CAD build for the part. Positions are in the model's coordinates, mm. A direction names the side the tool comes from. Give positions to 0.01 mm unless a question says otherwise; leave off trailing zeros. Write each loop counter-clockwise with the first axis right and the second up, starting at its lowest first coordinate (ties: lowest second). Pieces come first, ordered by that corner, then holes. Notation, with made-up numbers: (8.25, 14.5) - (66.25, 14.5) arc R29 cw to (66.25, 46.5) - close; hole circle Ø7 at (10, -34). An arc over 180 degrees is marked (long way). Answer as a JSON object with one key per item and string values.
from build123d import *

# Parameters (mm, degrees)
FLANGE_BASE1_DEPTH    = 5
CORTE_EXTRUS_O1_REACH = 55.903
ESBO_O2_R             = 1
QUEBRA_CANTO1_START   = -5
QUEBRA_CANTO1_DEPTH   = 5


# Read off the part's stored shape, not the designer's step: Quebra-Canto1
# Sheet-metal steps are written as plain solids
with BuildPart() as part:
    # Esboço1 → Flange-base1 (new body)
    with BuildSketch(Plane.XY):
        Polygon((-7.191672609, 43.102851176), (1.806254311, 43.102851176), (1.806254311, 37.302851176), (0.606254311, 37.302851176), (0.606254311, 34.902851176), (1.806254311, 34.902851176), (1.806254311, 31.102851176), (4.806254311, 31.102851176), (4.806254311, 34.902851176), (6.006254311, 34.902851176), (6.006254311, 37.302851176), (4.806254311, 37.302851176), (4.806254311, 43.102851176), (13.804181231, 43.102851176), (13.804181231, 48.102851176), (23.804181231, 48.102851176), (23.804181231, -21.897149822), (13.804181231, -21.897149822), (13.804181231, -16.897149822), (4.806254311, -16.897149822), (4.806254311, -11.097149822), (6.006254311, -11.097149822), (6.006254311, -8.697149822), (4.806254311, -8.697149822), (4.806254311, -4.897149822), (1.806254311, -4.897149822), (1.806254311, -8.697149822), (0.606254311, -8.697149822), (0.606254311, -11.097149822), (1.806254311, -11.097149822), (1.806254311, -16.897149822), (-7.191672609, -16.897149822), (-7.191672609, -21.897149822), (-17.191672609, -21.897149822), (-17.191672609, 48.10285125), (-7.191672609, 48.10285125), align=None)
    extrude(amount=-FLANGE_BASE1_DEPTH)

    # Esboço2 → Corte-extrusão1 (cut, up to next)
    with BuildSketch(Plane.XY, mode=Mode.PRIVATE) as corte_extrus_o1_sk1:
        with Locations((-7.191672609, 43.102851176)):
            Circle(ESBO_O2_R)
    corte_extrus_o1_tool1 = extrude(corte_extrus_o1_sk1.sketch, amount=-CORTE_EXTRUS_O1_REACH, mode=Mode.PRIVATE) & part.part
    # Esboço2 → Corte-extrusão1 (cut, up to next)
    with BuildSketch(Plane.XY, mode=Mode.PRIVATE) as corte_extrus_o1_sk2:
        with Locations((13.804181231, 43.102851176)):
            Circle(ESBO_O2_R)
    corte_extrus_o1_tool2 = extrude(corte_extrus_o1_sk2.sketch, amount=-CORTE_EXTRUS_O1_REACH, mode=Mode.PRIVATE) & part.part
    # Esboço2 → Corte-extrusão1 (cut, up to next)
    with BuildSketch(Plane.XY, mode=Mode.PRIVATE) as corte_extrus_o1_sk3:
        with Locations((13.804181231, -16.897149822)):
            Circle(ESBO_O2_R)
    corte_extrus_o1_tool3 = extrude(corte_extrus_o1_sk3.sketch, amount=-CORTE_EXTRUS_O1_REACH, mode=Mode.PRIVATE) & part.part
    # Esboço2 → Corte-extrusão1 (cut, up to next)
    with BuildSketch(Plane.XY, mode=Mode.PRIVATE) as corte_extrus_o1_sk4:
        with Locations((-7.191672609, -16.897149822)):
            Circle(ESBO_O2_R)
    corte_extrus_o1_tool4 = extrude(corte_extrus_o1_sk4.sketch, amount=-CORTE_EXTRUS_O1_REACH, mode=Mode.PRIVATE) & part.part
    add(corte_extrus_o1_tool1.solids().sort_by_distance((-7.191673, 43.102851, 0))[0], mode=Mode.SUBTRACT)
    add(corte_extrus_o1_tool2.solids().sort_by_distance((13.804181, 43.102851, 0))[0], mode=Mode.SUBTRACT)
    add(corte_extrus_o1_tool3.solids().sort_by_distance((13.804181, -16.89715, 0))[0], mode=Mode.SUBTRACT)
    add(corte_extrus_o1_tool4.solids().sort_by_distance((-7.191673, -16.89715, 0))[0], mode=Mode.SUBTRACT)

    # Quebra-Canto1 outline → Quebra-Canto1 (add)
    with BuildSketch(Plane.XY.offset(QUEBRA_CANTO1_START)):
        with BuildLine():
            Line((1.806254311, -4.897149822), (1.806254311, -5.897149822))
            ThreePointArc((1.806254311, -5.897149822), (2.09914753, -5.190043041), (2.806254311, -4.897149822))
            Line((2.806254311, -4.897149822), (1.806254311, -4.897149822))
        make_face()
        with BuildLine():
            Line((4.806254311, -4.897149822), (3.806254311, -4.897149822))
            ThreePointArc((3.806254311, -4.897149822), (4.513361092, -5.190043041), (4.806254311, -5.897149822))
            Line((4.806254311, -5.897149822), (4.806254311, -4.897149822))
        make_face()
        with BuildLine():
            Line((4.806254311, 31.102851176), (4.806254311, 32.102851176))
            ThreePointArc((4.806254311, 32.102851176), (4.513361092, 31.395744395), (3.806254311, 31.102851176))
            Line((3.806254311, 31.102851176), (4.806254311, 31.102851176))
        make_face()
        with BuildLine():
            Line((1.806254311, 31.102851176), (2.806254311, 31.102851176))
            ThreePointArc((2.806254311, 31.102851176), (2.09914753, 31.395744395), (1.806254311, 32.102851176))
            Line((1.806254311, 32.102851176), (1.806254311, 31.102851176))
        make_face()
    extrude(amount=QUEBRA_CANTO1_DEPTH)


solid = part.part
Item 1: Cut at A-A (y = 38). Give the cut face in (x, z).
Entries:
{"outline": "(-17.19, -5) - (1.81, -5) - (1.81, 0) - (-17.19, 0) - close; (4.81, -5) - (23.8, -5) - (23.8, 0) - (4.81, 0) - close"}
Item 2: Flat gauge pins, fed straight in: P1, Ø0.5, axis at x = 3.5, z = -1.5, coming from the -Y side; P2, Ø0.6, axis at x = 5, z = -3.5, coming from the +Y side. Where does each tip first touch, or does it go through?
Entries:
{"P1": "y = -4.9", "P2": "y = 43.1"}
Item 3: Which spindle directions (+Z, -Z, +X, -X, +Y, -Y) get a long thin tool onto all of the face, cutting with end or side? Do faces 1 (the flat face through (9, -16.897, -2)), 2 (the flat face through (6.006, -10, -2)), 3 (the flat face through (-7.192, 46, -2)). Say none if no direction does.
Entries:
{"face 1": "+Z, -Z, -Y", "face 2": "+Z, -Z", "face 3": "+Z, -Z, +Y"}
Item 4: Probe line 1 (X direction, y = 35.5, z = -0.5); line 2 (X direction, y = -12, z = -0.6); line 3 (Y direction, x = 14, z = -0.95). List the from-to ranges inside material, lowest first. Write a range as from..to.
Entries:
{"line 1": "-17.19..0.61, 6.01..23.8", "line 2": "-17.19..1.81, 4.81..23.8", "line 3": "-21.9..-17.88, -15.92..42.12, 44.08..48.1"}
Item 5: Mould opens along X. For faces 4 (the flat face through (-7.192, -20, -2)), 5 (the flat face through (19, 48.103, -2)) say: +X half, -X half, draft (parallel to the pull), parting line (faces both ways), or undercut.
Entries:
{"face 4": "undercut", "face 5": "draft"}
Item 6: Cut at B-B (x = -5). Give the cut face in (y, z).
Entries:
{"outline": "(-16.9, -5) - (43.1, -5) - (43.1, 0) - (-16.9, 0) - close"}
